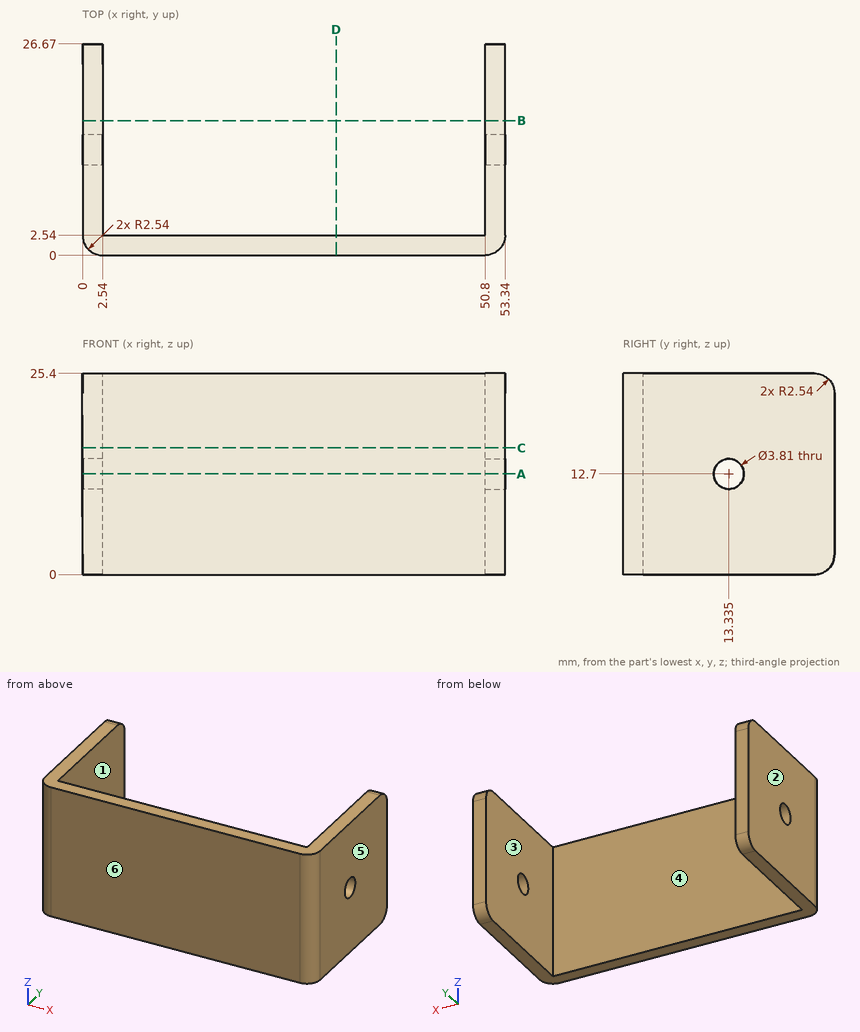
Can you work these out from the drawing? Everything is in mm from the part's minimum corner. A direction names the side the tool comes from. Coordinates: 2 decimals unless noted, no trailing zeros. Order: outer loops, then holes, each group sorted by start corner. A loop starts at its lowest first (then second) coordinate and runs counter-clockwise, first axis right, second up. Notation, with made-up numbers: (36.5, 16) -> (51.5, 16) arc R27 cw to (51.5, 42) -> close; hole circle Ø8 at (-20, -18.5). An arc over 180 degrees is marked (long way). Return JSON: item names as keys, results as strings.
1) If we section it at C-C on z = 16: List the corners of the cut face in (x, y) for me, plus the area to 3 significant figures.
Conclusion:
{"outline": "(0, 2.54) arc R2.54 ccw to (2.54, 0) -> (50.8, 0) arc R2.54 ccw to (53.34, 2.54) -> (53.34, 26.67) -> (50.8, 26.67) -> (50.8, 2.54) -> (2.54, 2.54) -> (2.54, 26.67) -> (0, 26.67) -> close", "area": "255 mm²"}
2) If we section it at B-B on y = 17: List the corners of the cut face in (x, z) for me, plus the area to 3 significant figures.
Conclusion:
{"outline": "(0, 0) -> (2.54, 0) -> (2.54, 25.4) -> (0, 25.4) -> close; (50.8, 0) -> (53.34, 0) -> (53.34, 25.4) -> (50.8, 25.4) -> close", "area": "129 mm²"}
3) I'm going to push a flat-ended pin straight in: P1, Ø7.5, axis at x = 21.5, z = 7, coming from the +Y side. Where does the tip first touch, or does it pass through?
Conclusion:
{"P1": "stops at y = 2.54"}
4) If I drill on probe 1 along X at (y, z) = (20, 18); probe 2 along Y at (x, z) = (37.5, 22.25), over which ranges is the centre line in solid material (lowest first)?
Conclusion:
{"probe 1": "x = 0 to 2.54, 50.8 to 53.34", "probe 2": "y = 0 to 2.54"}
5) If we section it at A-A on z = 12.7: List the corners of the cut face in (x, y) for me.
Conclusion:
{"outline": "(0, 2.54) arc R2.54 ccw to (2.54, 0) -> (50.8, 0) arc R2.54 ccw to (53.34, 2.54) -> (53.34, 11.43) -> (50.8, 11.43) -> (50.8, 2.54) -> (2.54, 2.54) -> (2.54, 11.43) -> (0, 11.43) -> close; (0, 15.24) -> (2.54, 15.24) -> (2.54, 26.67) -> (0, 26.67) -> close; (50.8, 15.24) -> (53.34, 15.24) -> (53.34, 26.67) -> (50.8, 26.67) -> close"}
6) If we section it at D-D on x = 32: List the corners of the cut face in (y, z) for me.
Conclusion:
{"outline": "(0, 0) -> (2.54, 0) -> (2.54, 25.4) -> (0, 25.4) -> close"}
7) Thinking about a two-plate mould opening in X: for the marked faces 3, 4, 5 and 6, which applies, +X half, -X half, draft (parallel to the pull), parting line (faces both ways), or undercut?
Conclusion:
{"face 3": "undercut", "face 4": "undercut", "face 5": "+X half", "face 6": "draft"}
8) On a 3-axis mill with a long thin cutter (end or side, diameter ignored), from which of +Z, -Z, +X, -X, +Y, -Y can I reach the whole of each face in a straight line? I mean the marked faces 1 and 2. Say none if no direction works.
Conclusion:
{"face 1": "+Z, -Z, +Y", "face 2": "+Z, -Z, -X, +Y, -Y"}
